Can you work these out from the drawing? Everything is in mm from the part's minimum corner. A direction names the side the tool comes from. Give positions to 0.01 mm unless a question says otherwise; leave off trailing zeros. Loops run counter-clockwise (first coordinate to the right, second up) from the corner with the lowest first, then second, coordinate; pieces in that order, holes last.
Q1. If we section it at D-D (y = 7.25): Please give me the cut outline in (x, z).
Q2. We'd pull the mould along X, two halves only. Please class the marked faces 1, 2 and 3: +X half, -X half, draft (parallel to the pull), parting line (faces both ways), or undercut.
Q3. I need wall thicknesses on line 1 (Y direction, x = 5, z = 3.95); line 2 (Z direction, x = 8, y = 5.5); line 3 (Y direction, x = 4, z = 2.5). Which ranges of each line are inside material? Lowest first, please.
Q4. If we section it at C-C (z = 2.35): Please give me the cut outline in (x, y).
Q5. If we section it at A-A (x = 5): Please give me the cut outline in (y, z), plus the area to 3 significant figures.
Q6. For the marked faces 4 and 5, which set-ups out of +Z, -Z, +X, -X, +Y, -Y let a thin tool reach every point of the face, with its end or its side?
Q7. Will these pins go through, and if not, where does the flat tip stop? P1, Ø1.5, axis at y = 8.5, z = 2, coming from the -X side; P2, Ø1, axis at x = 6, z = 1, coming from the +Y side.
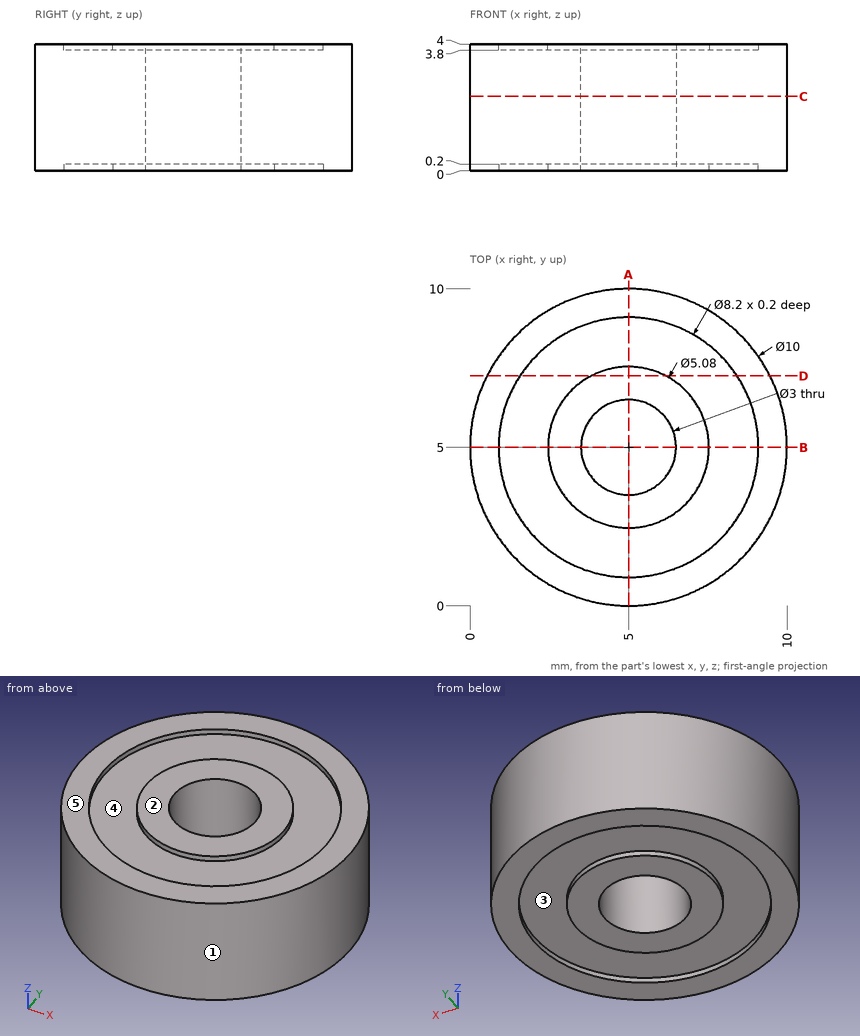
Check sheet entries:
1. outline: (0.53, 0) - (1.57, 0) - (1.57, 0.2) - (3.82, 0.2) - (3.82, 0) - (6.18, 0) - (6.18, 0.2) - (8.43, 0.2) - (8.43, 0) - (9.47, 0) - (9.47, 4) - (8.43, 4) - (8.43, 3.8) - (6.18, 3.8) - (6.18, 4) - (3.82, 4) - (3.82, 3.8) - (1.57, 3.8) - (1.57, 4) - (0.53, 4) - close
2. face 1: parting line
2. face 2: draft
2. face 3: undercut
3. line 1: y = 0 to 0.9, 2.46 to 3.5, 6.5 to 7.54, 9.1 to 10
3. line 2: z = 0.2 to 3.8
3. line 3: y = 0.1 to 3.88, 6.12 to 9.9
4. outline: circle Ø10 at (5, 5); hole circle Ø3 at (5, 5)
5. outline: (0, 0) - (0.9, 0) - (0.9, 0.2) - (2.46, 0.2) - (2.46, 0) - (3.5, 0) - (3.5, 4) - (2.46, 4) - (2.46, 3.8) - (0.9, 3.8) - (0.9, 4) - (0, 4) - close; (6.5, 0) - (7.54, 0) - (7.54, 0.2) - (9.1, 0.2) - (9.1, 0) - (10, 0) - (10, 4) - (9.1, 4) - (9.1, 3.8) - (7.54, 3.8) - (7.54, 4) - (6.5, 4) - close
5. area: 26.8 mm2
6. face 4: +Z
6. face 5: +Z, +X, -X, +Y, -Y
7. P1: stops at x = 0.82
7. P2: stops at y = 9.97
